from build123d import *


with BuildPart() as part:
    # 草图1 → 旋转1 (revolve)
    with BuildSketch(Plane.XY):
        with BuildLine():
            Line((0, 0), (20, 0))
            Line((20, 0), (30, 0))
            Line((30, 0), (30, 60))
            Line((30, 60), (20, 77.5))
            Line((20, 77.5), (20, 155))
            ThreePointArc((20, 155), (0, 163.284271247), (-20, 155))
            Line((-20, 155), (-20, 77.5))
            Line((-20, 77.5), (-30, 60))
            Line((-30, 60), (-30, 8))
            Line((-30, 8), (-50, 8))
            Line((-50, 8), (-50, 0))
            Line((-50, 0), (-30, 0))
            Line((-30, 0), (-20, 0))
            Line((-20, 0), (0, 0))
        make_face()
    revolve(axis=Axis((0, 0, 0), (-1, 0, 0)))


solid = part.part
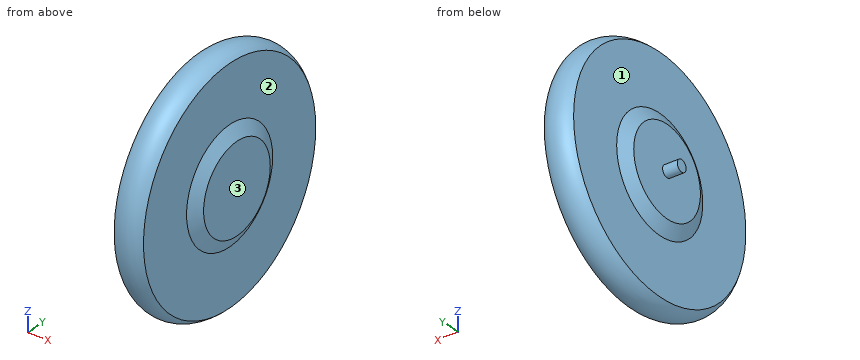
Could you check a few things on this model? Use its own coordinates, in mm. Face numbers are marked on the shaded views. A direction names the side the tool comes from. Round coordinates to 2 decimals unless told otherwise and drop trailing zeros. Order: outer loops, then holes, each group sorted by start corner. A loop starts at its lowest first (then second) coordinate and runs counter-clockwise, first axis right, second up.
(1) I'm going to push flat-ended pins straight in: pin 1 (10 mm diameter, centred on y = 101, z = -21, fed in from +X); pin 2 (3 mm diameter, centred on y = -36, z = -68, fed in from -X); pin 3 (4 mm diameter, centred on x = -8.5, z = 6, fed in from +Y). Where does each tip first touch, or does it pass through?
Response values:
pin 1: stops at x = 20
pin 2: stops at x = -21.18
pin 3: stops at y = 162.42
(2) Which directions (+Z, -Z, +X, -X, +Y, -Y) give clear straight access to the entire face, cutting with the end or side of a thin tool? Please do the marked faces 1, 2 and 3.
Response values:
face 1: -X
face 2: +X
face 3: +Z, -Z, +X, +Y, -Y
(3) Imagine slicing it at A-A (y = 0). Write out the boundary of the cut face in (x, z).
Response values:
outline: (-50, -8) - (-30, -8) - (-30, -60) - (-20, -77.5) - (-20, -155) arc R28.28 ccw to (20, -155) - (20, -77.5) - (30, -60) - (30, 60) - (20, 77.5) - (20, 155) arc R28.28 ccw to (-20, 155) - (-20, 77.5) - (-30, 60) - (-30, 8) - (-50, 8) - close
(4) Imagine slicing it at C-C (x = -1.5). Write out the boundary of the cut face in (y, z).
Response values:
outline: circle Ø326.49 at (0, 0)
(5) Imagine slicing it at D-D (x = 16). Write out the boundary of the cut face in (y, z), plus the area to 3 significant figures.
Response values:
outline: circle Ø316.65 at (0, 0)
area: 78,700 mm2
(6) Please list where these lines run through material, in increasing order: line 1 along X through (y, z) = (38, -74); line 2 along X through (y, z) = (-12, -53); line 3 along Z through (x, y) = (17, -51).
Response values:
line 1: x = -20 to 20
line 2: x = -30 to 30
line 3: z = -149.13 to 149.13
